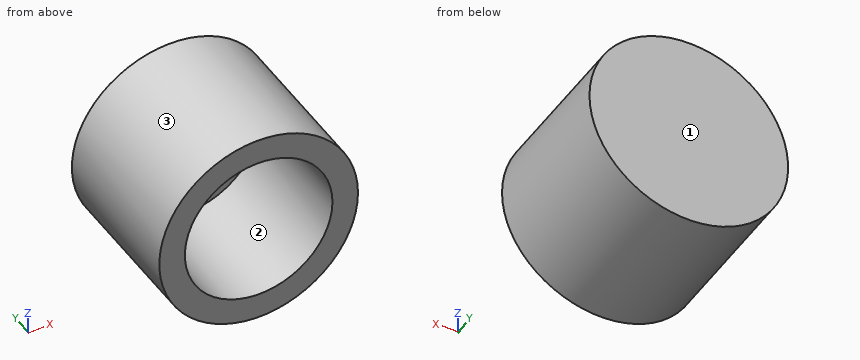
from build123d import *

# Parameters (mm, degrees)
F0_R     = 49.396191
F1_DEPTH = 76.2
F2_R     = 23.861127
F3_DEPTH = 50.8
F4_T     = -12.7


with BuildPart() as f1:
    # F0 (on Front) → F1 (new body)
    with BuildSketch(Plane.XZ):
        Circle(F0_R)
    extrude(amount=F1_DEPTH)

    # F2 (on Front) → F3 (join)
    with BuildSketch(Plane.XZ):
        Circle(F2_R)
    extrude(amount=F3_DEPTH)

    # F4
    f4_openings = [f1.faces().sort_by_distance(p)[0] for p in [
        (0, -76.2, 0),
    ]]
    offset(amount=F4_T, openings=f4_openings)


solid = f1.part
The model under review builds one solid part; all positions refer to its coordinate system, in mm. Face numbers are marked on the shaded views. Round coordinates to 2 decimals unless told otherwise and drop trailing zeros. Order: outer loops, then holes, each group sorted by start corner. A loop starts at its lowest first (then second) coordinate and runs counter-clockwise, first axis right, second up. Notation, with made-up numbers: (-10, 3) -> (37, 3) arc R24 ccw to (37, 26) -> close; hole circle Ø2 at (-13, 52.25). An arc over 180 degrees is marked (long way). Return JSON: item names as keys, results as strings.
1. The part is to be moulded in two halves that separate along Z. For the marked faces 1, 2 and 3, say which applies: +Z half, -Z half, draft (parallel to the pull), parting line (faces both ways), or undercut.
Answer block:
{"face 1": "draft", "face 2": "undercut", "face 3": "parting line"}
2. Take a section at D-D (x = -38). Write out the cut boundary in (y, z), then the cut area to 3 significant figures.
Answer block:
{"outline": "(-76.2, -31.56) -> (0, -31.56) -> (0, 31.56) -> (-76.2, 31.56) -> close", "area": "4,810 mm²"}
3. Take a section at C-C (y = -17.5). Write out the cut boundary in (x, z).
Answer block:
{"outline": "circle Ø98.79 at (0, 0); hole circle Ø73.39 at (0, 0)"}
4. Take a section at B-B (z = 0). Write out the cut boundary in (x, y), then the cut area to 3 significant figures.
Answer block:
{"outline": "(-49.4, -76.2) -> (-36.7, -76.2) -> (-36.7, -12.7) -> (36.7, -12.7) -> (36.7, -76.2) -> (49.4, -76.2) -> (49.4, 0) -> (-49.4, 0) -> close", "area": "2,870 mm²"}
5. For L1, parallel to Z at x = 0, y = -51.5; L2, parallel to Y at x = 0.5, z = -19.5; L3, parallel to Z at x = 14.5, y = -44.5, list the stretches that pass through material, from the lowest coordinate up. Write a range as [from, to].
Answer block:
{"L1": "z = [-49.4, -36.7], [36.7, 49.4]", "L2": "y = [-12.7, 0]", "L3": "z = [-47.22, -33.71], [33.71, 47.22]"}
6. Insertion check: P1, Ø1.5, axis at x = -38.5, y = -43.5, coming from the -Z side; P2, Ø12, axis at y = -57, z = 2.5, coming from the -X side; P3, Ø22, axis at x = 14.5, z = 0.5, coming from the -Y side; P4, Ø1.5, axis at y = -31.5, z = 7, coming from the +X side. Each pin has a flat end and moves straight along its axis. Give the tip position at first contact, or say it passes through.
Answer block:
{"P1": "stops at z = -31.86", "P2": "stops at x = -49.4", "P3": "stops at y = -12.7", "P4": "stops at x = 49"}
7. Take a section at A-A (x = 0). Write out the cut boundary in (y, z).
Answer block:
{"outline": "(-76.2, -49.4) -> (0, -49.4) -> (0, 49.4) -> (-76.2, 49.4) -> (-76.2, 36.7) -> (-12.7, 36.7) -> (-12.7, -36.7) -> (-76.2, -36.7) -> close"}
